Input: dimensioned drawing with shaded views. Units: mm. Origin: part minimum x, y, z. Round coordinates to 2 decimals unless told otherwise and drop trailing zeros. Loops run counter-clockwise (first coordinate to the right, second up) from the corner with the lowest first, then second, coordinate; pieces in that order, holes last.
Item 1: Ray query, L1, parallel to Y at x = 56, z = 6.5; L2, parallel to X at y = 45, z = 4; L3, parallel to Y at x = 41.5, z = 8.25. Return the intervals inside material, ascending.
Item 2: Section query D-D on y = 39.5. Return loops of the section in (x, z).
Item 3: First-contact query: P1, Ø3.5, axis at x = 25.36, y = 4, coming from the +Z side; P2, Ø1.5, axis at x = 73, z = 1, coming from the +Y side. Flat tips, straight axial feed; report the tip coordinate or a pass-through.
Item 4: Section query B-B on z = 4. Return loops of the section in (x, y) (1 decimal).
Item 5: Section query A-A on y = 4. Return loops of the section in (x, z) (1 decimal), then the cut area to 3 significant figures.
Item 6: Section query C-C on x = 55.5. Return loops of the section in (y, z), then the cut area to 3 significant figures.
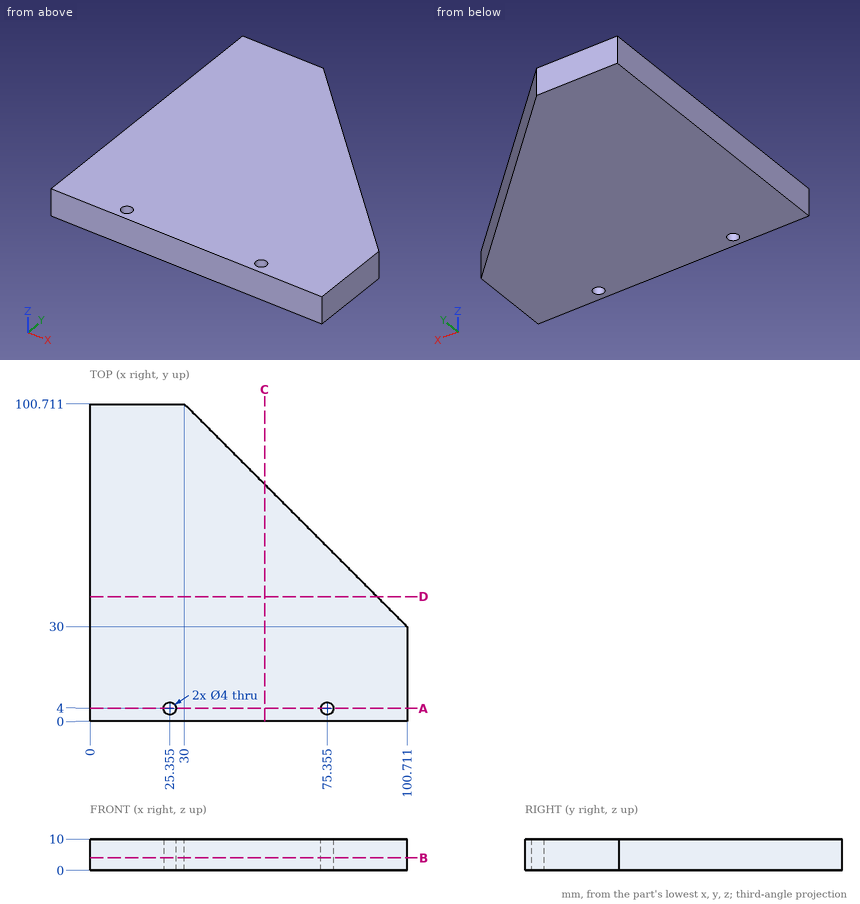
Data:
1. L1: y = 0 to 74.71
1. L2: x = 0 to 85.71
1. L3: y = 0 to 89.21
2. outline: (0, 0) - (91.21, 0) - (91.21, 10) - (0, 10) - close
3. P1: passes through
3. P2: stops at y = 58.46
4. outline: (0, 0) - (100.7, 0) - (100.7, 30) - (30, 100.7) - (0, 100.7) - close; hole circle Ø4 at (25.4, 4); hole circle Ø4 at (75.4, 4)
5. outline: (0, 0) - (23.4, 0) - (23.4, 10) - (0, 10) - close; (27.4, 0) - (73.4, 0) - (73.4, 10) - (27.4, 10) - close; (77.4, 0) - (100.7, 0) - (100.7, 10) - (77.4, 10) - close
5. area: 927 mm2
6. outline: (0, 0) - (75.21, 0) - (75.21, 10) - (0, 10) - close
6. area: 752 mm2
